Work out the finished part from the listing and answer in its coordinate system (mm). Face numbers are marked on the shaded views. A direction names the side the tool comes from. Give positions to 0.01 mm unless a question says otherwise; leave off trailing zeros. Write each loop counter-clockwise with the first axis right and the second up, starting at its lowest first coordinate (ties: lowest second). Pieces come first, ordered by that corner, then holes.
1) Find section C-C (z = 24.5). Determine the outline of the cut face in (x, y), plus the area to 3 significant figures.
2) A tool of negligible diameter and unlimited length cuts with its end or side. For the marked faces 1, 2 and 3, from which of +Z, -Z, +X, -X, +Y, -Y can it reach the whole face along a straight path? Write none if from no direction.
3) Straight lines are drawn through the part: probe 1 along Y at (x, z) = (0, 33); probe 2 along X at (y, z) = (6, 13); probe 3 along Z at (x, y) = (-12, 19). For each, find the intervals that lie inside material, in ascending order.
4) Find section D-D (z = 1). Determine the outline of the cut face in (x, y).
5) Given pin 1 Ø4.5 at (x, y) = (-10.5, 11) entering from -Z; pin 2 Ø1 at (x, z) = (17, 25.5) entering from +Y; pin 3 Ø5 at (x, y) = (0, 0) entering from -Z, each flat-ended and moving along its own axis, determine where each tip first touches the part or whether it passes through.
6) Determine the mould class of the marked faces 4, 5 and 6 for opening direction Y: pulls with the +Y half, pulls with the -Y half, needs draft (parallel to the pull), parting line crosses it, or undercut.
7) Find section B-B (y = -20). Determine the outline of the cut face in (x, z), plus the area to 3 significant figures.
8) Find section A-A (z = 30). Determine the outline of the cut face in (x, y), plus the area to 3 significant figures.
```python
from build123d import *

# Parameters (mm, degrees)
SKETCH1_R           = 19
BOSS_EXTRUDE1_DEPTH = 26
SKETCH2_R           = 10
BOSS_EXTRUDE2_DEPTH = 3
SKETCH3_R           = 6
BOSS_EXTRUDE3_DEPTH = 12
SKETCH4_R           = 4
CUT_EXTRUDE1_DEPTH  = 10
SKETCH5_R           = 4
BOSS_EXTRUDE4_DEPTH = 24
FILLET1_R           = 4
BOSS_EXTRUDE5_DEPTH = 6
CUT_EXTRUDE2_REACH  = 57.794
FILLET2_R           = 2
FILLET3_R           = 2


with BuildPart() as part:
    # Sketch1 → Boss-Extrude1 (new body)
    with BuildSketch(Plane.XY):
        with Locations(Location((0, 0, 0), (0, 0, 180))):
            Circle(SKETCH1_R)
    extrude(amount=BOSS_EXTRUDE1_DEPTH)

    # Sketch2 → Boss-Extrude2 (add)
    with BuildSketch(Plane.XY.offset(26)):
        Circle(SKETCH2_R)
    extrude(amount=BOSS_EXTRUDE2_DEPTH)

    # Sketch3 → Boss-Extrude3 (add)
    with BuildSketch(Plane.XY.offset(29)):
        Circle(SKETCH3_R)
    extrude(amount=BOSS_EXTRUDE3_DEPTH)

    # Sketch4 → Cut-Extrude1 (cut)
    with BuildSketch(Plane.XY.offset(41)):
        Circle(SKETCH4_R)
    extrude(amount=-CUT_EXTRUDE1_DEPTH, mode=Mode.SUBTRACT)

    # Sketch5 → Boss-Extrude4 (add)
    with BuildSketch(Plane(origin=(0, 0, 0), x_dir=(1, 0, 0), z_dir=(0, 1, 0))):
        with Locations(Location((0, 0, 0), (0, 0, 270))):
            Circle(SKETCH5_R)
    extrude(amount=-BOSS_EXTRUDE4_DEPTH)

    # Fillet1
    fillet1_edges = [part.edges().sort_by_distance(p)[0] for p in [
        (0, 0, -4),
    ]]
    fillet(fillet1_edges, radius=FILLET1_R - 0.0001)  # a hair under: the kernel refuses the full size

    # Sketch6 → Boss-Extrude5 (add, symmetric)
    with BuildSketch(Plane(origin=(0, 0, 0), x_dir=(-0.7071067811865464, 0.7071067811865488, 0), z_dir=(0.7071067811865488, 0.7071067811865464, 0))):
        with BuildLine():
            Line((-14.845299462, 26), (-10.515172443, 33.5))
            ThreePointArc((-10.515172443, 33.5), (-10.515172443, 38.5), (-14.845299462, 41))
            Line((-14.845299462, 41), (-26, 41))
            Line((-26, 41), (-26, 40))
            Line((-26, 40), (-14.845299462, 40))
            ThreePointArc((-14.845299462, 40), (-11.381197846, 38), (-11.381197846, 34))
            Line((-11.381197846, 34), (-16, 26))
            Line((-16, 26), (-14.845299462, 26))
        make_face()
        with BuildLine():
            Line((26, 41), (26, 40))
            Line((26, 40), (14.845299462, 40))
            ThreePointArc((14.845299462, 40), (11.381197846, 38), (11.381197846, 34))
            Line((11.381197846, 34), (16, 26))
            Line((16, 26), (14.845299462, 26))
            Line((14.845299462, 26), (10.515172443, 33.5))
            ThreePointArc((10.515172443, 33.5), (10.515172443, 38.5), (14.845299462, 41))
            Line((14.845299462, 41), (26, 41))
        make_face()
    extrude(amount=BOSS_EXTRUDE5_DEPTH, both=True)

    # Sketch7 → Cut-Extrude2 (cut, up to next)
    with BuildSketch(Plane.XY.offset(41), mode=Mode.PRIVATE) as cut_extrude2_sk1:
        with BuildLine():
            Line((-18.03122292, 16.334166645), (-16.334166645, 18.03122292))
            ThreePointArc((-16.334166645, 18.03122292), (-13.788582233, 18.03122292), (-13.788582233, 15.485638508))
            Line((-13.788582233, 15.485638508), (-15.485638508, 13.788582233))
            ThreePointArc((-15.485638508, 13.788582233), (-18.03122292, 13.788582233), (-18.03122292, 16.334166645))
        make_face()
    cut_extrude2_tool1 = extrude(cut_extrude2_sk1.sketch, amount=-CUT_EXTRUDE2_REACH, mode=Mode.PRIVATE) & part.part
    # Sketch7 → Cut-Extrude2 (cut, up to next)
    with BuildSketch(Plane.XY.offset(41), mode=Mode.PRIVATE) as cut_extrude2_sk2:
        with BuildLine():
            Line((15.485638508, -13.788582233), (13.788582233, -15.485638508))
            ThreePointArc((13.788582233, -15.485638508), (13.788582233, -18.03122292), (16.334166645, -18.03122292))
            Line((16.334166645, -18.03122292), (18.03122292, -16.334166645))
            ThreePointArc((18.03122292, -16.334166645), (18.03122292, -13.788582233), (15.485638508, -13.788582233))
        make_face()
    cut_extrude2_tool2 = extrude(cut_extrude2_sk2.sketch, amount=-CUT_EXTRUDE2_REACH, mode=Mode.PRIVATE) & part.part
    add(cut_extrude2_tool1.solids().sort_by_distance((-15.909903, 15.909903, 41))[0], mode=Mode.SUBTRACT)
    add(cut_extrude2_tool2.solids().sort_by_distance((15.909903, -15.909903, 41))[0], mode=Mode.SUBTRACT)

    # Fillet2
    fillet2_edges = [part.edges().sort_by_distance(p)[0] for p in [
        (14.142135624, -22.627416998, 40.5),
        (22.627416998, -14.142135624, 40.5),
        (-22.627416998, 14.142135624, 40.5),
        (-14.142135624, 22.627416998, 40.5),
    ]]
    fillet(fillet2_edges, radius=FILLET2_R)

    # Fillet3
    fillet3_edges = [part.edges().sort_by_distance(p)[0] for p in [
        (11.313708499, -11.313708499, 26),
        (-11.313708499, 11.313708499, 26),
    ]]
    fillet(fillet3_edges, radius=FILLET3_R)


solid = part.part
```
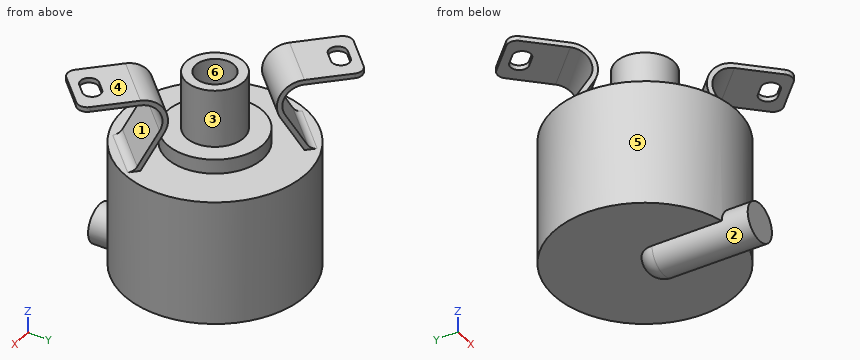
Results:
1. outline: circle Ø38 at (0, 0)
1. area: 1,130 mm2
2. face 1: +X, -Y
2. face 2: -Y
2. face 3: +Z
3. probe 1: y = -6 to -4, 4 to 6
3. probe 2: x = -18.03 to 18.03
3. probe 3: z = 40 to 41
4. outline: (-3.87, -24) - (3.87, -24) - (3.87, -18.6) arc R19 ccw (long way) to (-3.87, -18.6) - close
5. pin 1: stops at z = 0
5. pin 2: stops at y = 9.42
5. pin 3: stops at z = -3.71
6. face 4: needs draft
6. face 5: parting line crosses it
6. face 6: undercut
7. outline: circle Ø8 at (0, 0); (11.51, 40) - (16.77, 40) - (16.77, 41) - (11.51, 41) - close
7. area: 55.5 mm2
8. outline: (-13.92, 5.44) - (-13.11, 4.62) - (-4.62, 13.11) - (-5.44, 13.92) - close; circle Ø12 at (0, 0); (4.62, -13.11) - (5.44, -13.92) - (13.92, -5.44) - (13.11, -4.62) - close
8. area: 141 mm2
